from build123d import *

# Parameters (mm, degrees)
SKETCH1_W           = 225
SKETCH1_H           = 173
BOSS_EXTRUDE1_DEPTH = 5
SKETCH2_W           = 9.9
SKETCH2_H           = 1.2
BOSS_EXTRUDE2_DEPTH = 5
SKETCH3_W           = 9.9
SKETCH3_H           = 1.2
BOSS_EXTRUDE3_DEPTH = 5


with BuildPart() as part:
    # Sketch1 → Boss-Extrude1 (new body)
    with BuildSketch(Plane(origin=(0, 0, 0), x_dir=(1, 0, 0), z_dir=(0, 1, 0))):
        with Locations((112.5, 86.5)):
            Rectangle(SKETCH1_W, SKETCH1_H)
    extrude(amount=BOSS_EXTRUDE1_DEPTH)

    # Sketch2 → Boss-Extrude2 (add)
    with BuildSketch(Plane.ZY):
        with Locations((-150.05, 2.15)):
            Rectangle(SKETCH2_W, SKETCH2_H)
        with Locations((-22.95, 2.15)):
            Rectangle(SKETCH2_W, SKETCH2_H)
    extrude(amount=BOSS_EXTRUDE2_DEPTH)

    # Sketch3 → Boss-Extrude3 (add)
    with BuildSketch(Plane(origin=(225, 0, 0), x_dir=(0, 0, -1), z_dir=(1, 0, 0))):
        with Locations((22.95, 2.15)):
            Rectangle(SKETCH3_W, SKETCH3_H)
        with Locations((150.05, 2.15)):
            Rectangle(SKETCH3_W, SKETCH3_H)
    extrude(amount=BOSS_EXTRUDE3_DEPTH)


solid = part.part
Work out the finished part from the listing and answer in its coordinate system (mm). A direction names the side the tool comes from. Round coordinates to 2 decimals unless told otherwise and drop trailing zeros. Write each loop counter-clockwise with the first axis right and the second up, starting at its lowest first coordinate (ties: lowest second). Pieces come first, ordered by that corner, then holes. Notation, with made-up numbers: M -34,12.5 L 18,12.5 A21 ccw 18,40.5 Z; hole C 2.5,76.25 d5. An arc over 180 degrees is marked long. Use a Markdown table: item, result.
1) Flat-ended cylindrical pins translate along their axes: pin 1 (4 mm diameter, centred on x = -2.5, z = -149, fed in from -Y); pin 2 (1.5 mm diameter, centred on y = 3, z = -54, fed in from +X); pin 3 (1.5 mm diameter, centred on x = 228.5, z = -22.5, fed in from +Y). Find the tip coordinate at first contact, or state that the pin passes through.
Taken from the geometry:
| item | result |
|---|---|
| pin 1 | stops at y = 1.55 |
| pin 2 | stops at x = 225 |
| pin 3 | stops at y = 2.75 |
2) Determine the mould class of faces 4 (the face through (111, 2, -173)), 5 (the face through (-2, 2.75, -23)), 6 (the face through (225, 2, -85)) for opening direction Z: pulls with the +Z half, pulls with the -Z half, needs draft (parallel to the pull), parting line crosses it, or undercut.
Taken from the geometry:
| item | result |
|---|---|
| face 4 | pulls with the -Z half |
| face 5 | needs draft |
| face 6 | undercut |
3) Consider line 1 (X direction, y = 3.1, z = -115). Determine where the line is inside the solid, lowest interval first. Write a range as [from, to].
Taken from the geometry:
| item | result |
|---|---|
| line 1 | x = [0, 225] |
4) The part is cut by section A-A on z = -127. Give the vertices of the cut face in (x, y).
Taken from the geometry:
| item | result |
|---|---|
| outline | M 0,0 L 225,0 L 225,5 L 0,5 Z |
5) Which of the six approach directions +Z, -Z, +X, -X, +Y, -Y give full straight-line access (tool end or side, diameter ignored) to faces 1 (the face through (-2, 2.75, -150)), 2 (the face through (227, 1.55, -150)), 3 (the face through (-2, 1.55, -23))?
Taken from the geometry:
| item | result |
|---|---|
| face 1 | +Z, -Z, -X, +Y |
| face 2 | +Z, -Z, +X, -Y |
| face 3 | +Z, -Z, -X, -Y |
